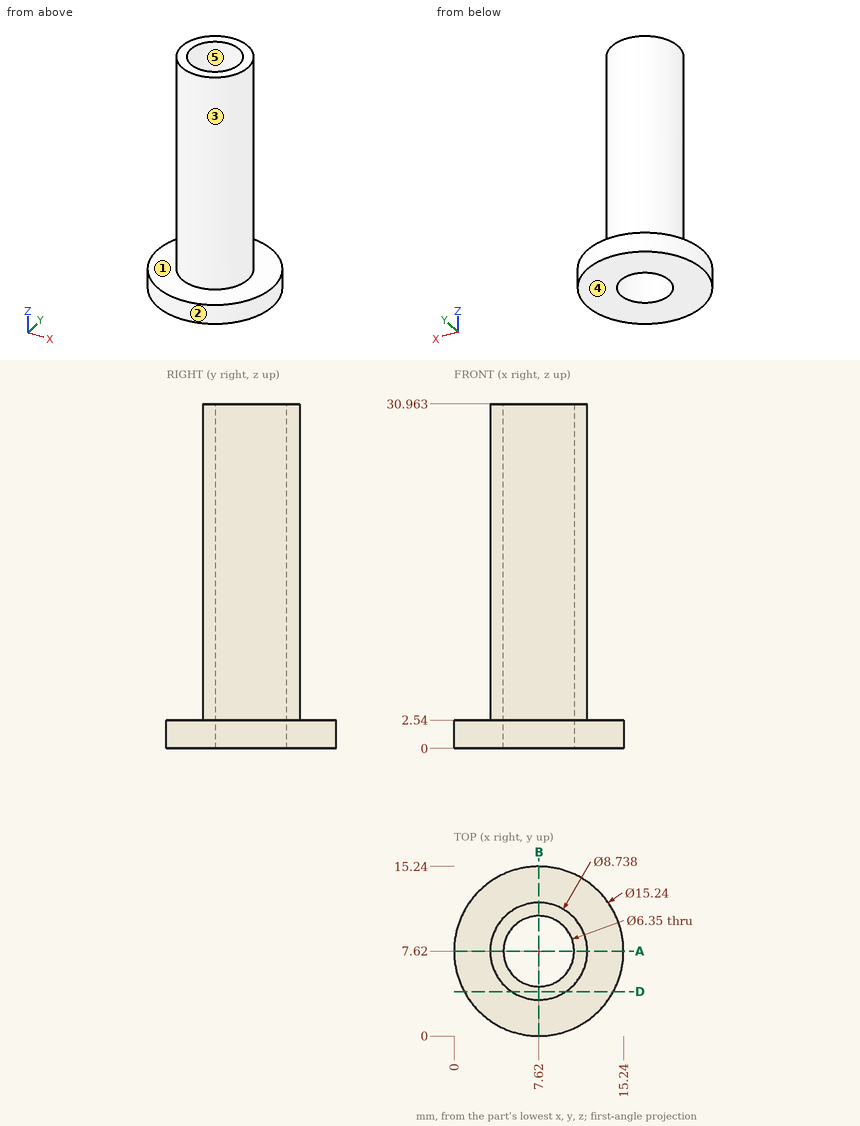
For this review, use the dimensioned drawing (mm, ordinates from the lowest corner) and the shaded views. A direction names the side the tool comes from. Round coordinates to 2 decimals unless told otherwise and drop trailing zeros. Write each loop counter-clockwise with the first axis right and the second up, starting at its lowest first coordinate (ties: lowest second). Pieces come first, ordered by that corner, then holes. Notation, with made-up numbers: M 28,59.25 L 86,59.25 A33 ccw 86,94.25 Z; hole C 81.25,-6.5 d1. An arc over 180 degrees is marked long. Answer as CSV lines item,"result". Start each with the question number.
Q1. Wall thickness on line 1 along Y through (x, z) = (7.62, 8.5) (1 decimal); line 2 along Z through (x, y) = (1.5, 8.25); line 3 along Y through (x, z) = (9, 24.5) (1 decimal): over which ranges is each line inside the solid? List them lowest first.
Q2. Consider section D-D, the plane y = 4. Give the boundary of the cut face in (x, z) (1 decimal).
Q3. Tool access review of the marked faces 1 and 2: name each direction out of +Z, -Z, +X, -X, +Y, -Y from which nothing blocks a thin tool from reaching the whole face with its end or side.
Q4. The part is to be moulded in two halves that separate along Y. For the marked faces 3, 4 and 5, say which applies: +Y half, -Y half, draft (parallel to the pull), parting line (faces both ways), or undercut.
Q5. Consider section A-A, the plane y = 7.62. Give the boundary of the cut face in (x, z) (1 decimal).
Q6. Clearance check with flat-ended pins moving along their axes: P1, Ø4, axis at x = 9, z = 19, coming from the +Y side; P2, Ø6, axis at y = 10, z = 25, coming from the -X side; P3, Ø5, axis at x = 9, z = 9.5, coming from the -Y side. State where each tip first meets the part, or that it passes through.
Result set:
1,line 1,"y = 3.3 to 4.4, 10.8 to 12"
1,line 2,"z = 0 to 2.54"
1,line 3,"y = 3.5 to 4.8, 10.5 to 11.8"
2,outline,"M 0.9,0 L 14.3,0 L 14.3,2.5 L 10.1,2.5 L 10.1,31 L 5.2,31 L 5.2,2.5 L 0.9,2.5 Z"
3,face 1,"+Z"
3,face 2,"+Z, -Z"
4,face 3,"parting line"
4,face 4,"draft"
4,face 5,"undercut"
5,outline,"M 0,0 L 4.4,0 L 4.4,31 L 3.3,31 L 3.3,2.5 L 0,2.5 Z; M 10.8,0 L 15.2,0 L 15.2,2.5 L 12,2.5 L 12,31 L 10.8,31 Z"
6,P1,"stops at y = 11.99"
6,P2,"stops at x = 3.25"
6,P3,"stops at y = 3.25"
